Design review of the part shown in the three views and the two pictorial views. Dimensions are in mm from the part's minimum x, y and z. A direction names the side the tool comes from. Round coordinates to 2 decimals unless told otherwise and drop trailing zeros. Loops run counter-clockwise (first coordinate to the right, second up) from the corner with the lowest first, then second, coordinate; pieces in that order, holes last. Notation, with made-up numbers: M -35.5,-39.75 L -2.5,-39.75 A13 cw -2.5,-32.75 Z; hole C 34,-31 d9. An arc over 180 degrees is marked long. One line per question, with ' | ' between items.
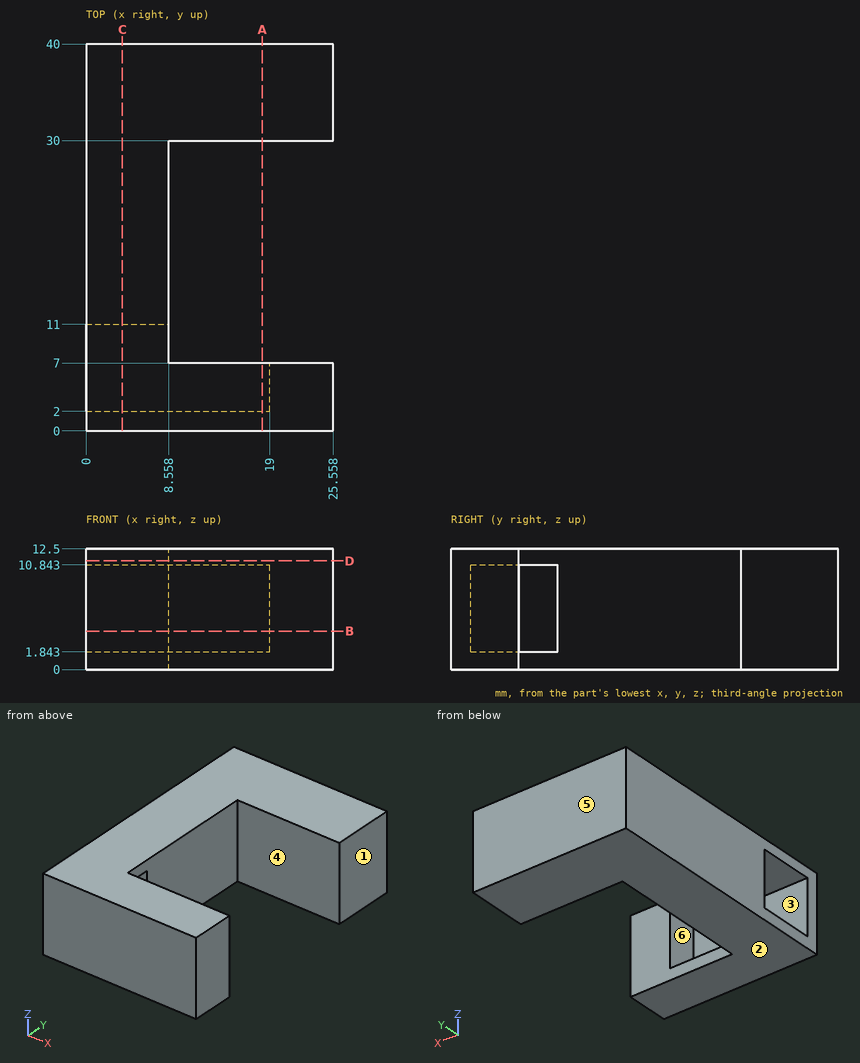
1) Mouldability with a two-part tool opening along Z and no side actions: class the marked faces 1, 2 and 3 as +Z half, -Z half, draft (parallel to the pull), parting line (faces both ways), or undercut.
Output values:
face 1: draft | face 2: -Z half | face 3: undercut
2) Machinability: for the marked faces 4, 5 and 6, which of the approach directions +Z, -Z, +X, -X, +Y, -Y give a long, thin tool a straight path to every point of the face, cutting with its end or side? Answer none if there is none.
Output values:
face 4: +Z, -Z, +X | face 5: +Z, -Z, +X, -X, +Y | face 6: -X
3) Insertion check: P1, Ø6, axis at x = 13.5, y = 20, coming from the +Z side; P2, Ø2.5, axis at y = 5, z = 6.5, coming from the -X side. Each pin has a flat end and moves straight along its axis. Give the tip position at first contact, or say it passes through.
Output values:
P1: passes through | P2: stops at x = 19
4) Add section A-A on x = 18.25. State the section outline as (y, z) points.
Output values:
outline: M 0,0 L 7,0 L 7,1.84 L 2,1.84 L 2,10.84 L 7,10.84 L 7,12.5 L 0,12.5 Z; M 30,0 L 40,0 L 40,12.5 L 30,12.5 Z
5) For line 1 (Y direction, x = 15.5, z = 10.75); line 2 (Y direction, x = 20.25, z = 7.25); line 3 (X direction, y = 21, z = 10.5), list the stretches that pass through material, from the lowest coordinate up.
Output values:
line 1: y = 0 to 2, 30 to 40 | line 2: y = 0 to 7, 30 to 40 | line 3: x = 0 to 8.56
6) Add section C-C on x = 3.75. State the section outline as (y, z) points, then the cut area to 3 significant figures.
Output values:
outline: M 0,0 L 40,0 L 40,12.5 L 0,12.5 Z; hole M 2,1.84 L 11,1.84 L 11,10.84 L 2,10.84 Z | area: 419 mm²
7) Add section D-D on z = 11.25. State the section outline as (x, y) points.
Output values:
outline: M 0,0 L 25.56,0 L 25.56,7 L 8.56,7 L 8.56,30 L 25.56,30 L 25.56,40 L 0,40 Z
8) Add section B-B on z = 4. State the section outline as (x, y) points, then the cut area to 3 significant figures.
Output values:
outline: M 0,0 L 25.56,0 L 25.56,7 L 19,7 L 19,2 L 0,2 Z; M 0,11 L 8.56,11 L 8.56,30 L 25.56,30 L 25.56,40 L 0,40 Z | area: 502 mm²
